Read the model definition and answer for the solid it produces. Units are mm, in the model's axes. Face numbers are marked on the shaded views. A direction names the side the tool comes from. Coordinates: 2 decimals unless noted, no trailing zeros. Write each loop counter-clockwise with the first axis right and the second up, starting at its lowest first coordinate (ties: lowest second). Pieces come first, ordered by that corner, then holes.
Item 1: Section A-A (x = -20) is taken. Give the vertices of the cut face in (y, z).
Item 2: This flat-tipped pin is pushed along its axis until it touches: P1, Ø1.5, axis at x = -9, y = -6.5, coming from the -Z side. Where does it stop, or does it pass through?
Item 3: Straight lines are drawn through the part: probe 1 along Z at (x, y) = (-14.5, -8.5); probe 2 along X at (y, z) = (-7, 20). For each, find the intervals that lie inside material, in ascending order.
Item 4: A tool of negligible diameter and unlimited length cuts with its end or side. For the marked faces 1 and 2, from which of +Z, -Z, +X, -X, +Y, -Y can it reach the whole face along a straight path? Write none if from no direction.
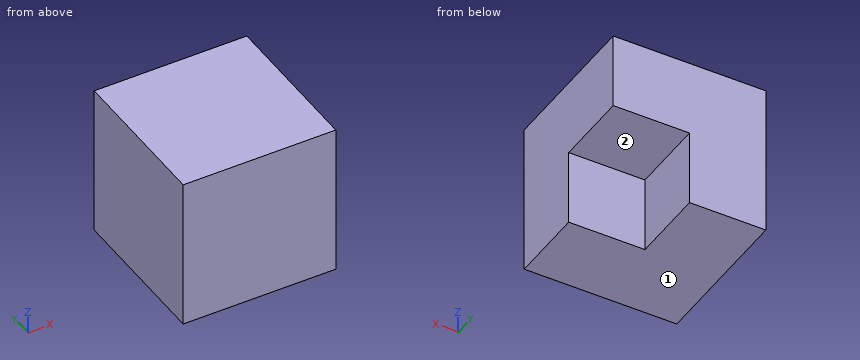
from build123d import *

# Parameters (mm, degrees)
F2_DEPTH = 50.8
F1_W     = 25.4
F1_H     = 25.4
F3_DEPTH = 25.4


with BuildPart() as f2:
    # F0 (on Front) → F2 (new body)
    with BuildSketch(Plane.XZ):
        Polygon((-25.4, 0), (0, 0), (0, 25.4), (0, 50.8), (-50.8, 50.8), (-50.8, 0), align=None)
    extrude(amount=F2_DEPTH)

    # F1 (on face) → F3 (cut)
    with BuildSketch(Plane.XZ):
        with Locations((-12.7, 12.7)):
            Rectangle(F1_W, F1_H)
    extrude(amount=F3_DEPTH, mode=Mode.SUBTRACT)


solid = f2.part
Established:
1. outline: (-50.8, 0) - (-25.4, 0) - (-25.4, 25.4) - (0, 25.4) - (0, 50.8) - (-50.8, 50.8) - close
2. P1: stops at z = 25.4
3. probe 1: z = 25.4 to 50.8
3. probe 2: x = -50.8 to -25.4
4. face 1: -Z, +X, -X, +Y, -Y
4. face 2: -Z, +X, +Y
